Verification items for the finished model (mm, model axes). Face numbers are marked on the shaded views. A direction names the side the tool comes from. Coordinates: 2 decimals unless noted, no trailing zeros. Loops run counter-clockwise (first coordinate to the right, second up) from the corner with the lowest first, then second, coordinate; pieces in that order, holes last. Notation, with made-up numbers: (45.25, -12.5) -> (64.25, -12.5) arc R8 ccw to (64.25, -3.5) -> close; hole circle Ø9 at (29, -40). An arc over 180 degrees is marked (long way). Answer as a JSON object with one key per item and string values. Group by question number.
Q1. Cross-section at B-B on z = -4.75. Record the boundary of the cut face in (x, y) (3 decimals).
Q2. Cross-section at C-C on z = -2.75. Record the boundary of the cut face in (x, y) (3 decimals), and give its area (3 significant figures).
Q3. Scan lines: L1, parallel to X at y = 0, z = 4.05 (3 decimals); L2, parallel to X at y = 0, z = 2.5 (3 decimals); L3, parallel to X at y = 0, z = -3.95 (3 decimals). Record each from-to range of solid material in increasing order.
Q4. Set-up check for the marked faces 1, 2 and 3: record each of +Z, -Z, +X, -X, +Y, -Y from which the full face is reachable in a straight line by a thin tool's end or side.
Q5. Gauge pin test, flat ends, axial feed: pin 1 Ø4 at (y, z) = (-6, 4) entering from -X; pin 2 Ø1 at (y, z) = (-6, 1.5) entering from -X; pin 3 Ø3 at (x, y) = (8.5, 8) entering from -Z. Record the tip position at first contact, or that the pin passes through.
Q6. Release check for a two-part mould opening along Y. For the marked faces 4, 5, 6 and 7 record: released by +Y, released by -Y, zero draft, split by the parting line, or undercut.
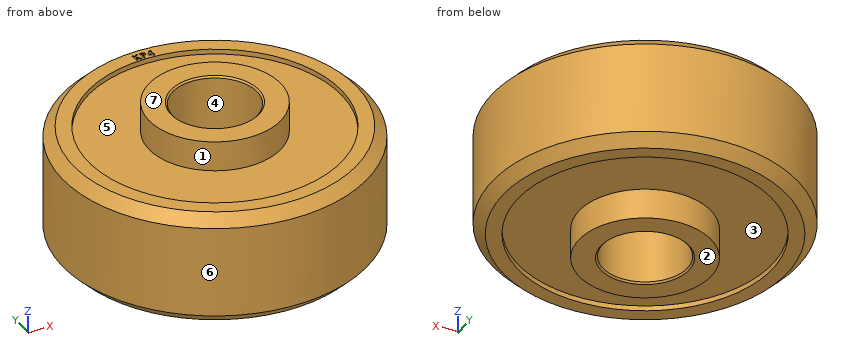
```python
from build123d import *

# Parameters (mm, degrees)
CUT_EXTRUDE1_DEPTH = 0.0635


with BuildPart() as part:
    # Sketch1 → Revolve1 (revolve)
    with BuildSketch(Plane(origin=(0, 0, 0), x_dir=(0, 0, -1), z_dir=(1, 0, 0))):
        Polygon((-6.1468, 3.302), (-6.1468, 4.953), (-3.8735, 4.953), (-3.8735, 9.525), (-4.2545, 9.525), (-4.2545, 10.63498), (-3.4417, 11.44778), (3.4417, 11.44778), (4.2545, 10.63498), (4.2545, 9.525), (3.8735, 9.525), (3.8735, 4.953), (6.1468, 4.953), (6.1468, 3.302), (6.0198, 3.175), (-6.0198, 3.175), align=None)
    revolve(axis=Axis((0, 0, 0), (0, 0, -1)))

    # Sketch2 → Cut-Extrude1 (cut)
    with BuildSketch(Plane.XY.offset(4.2545)):
        Polygon((-0.715797037, 10.256682265), (-0.59431767, 10.262024813), (-0.584777405, 10.044761191), (-0.422974521, 10.269529821), (-0.278344112, 10.275889997), (-0.486703487, 9.984593924), (-0.229243551, 9.645214917), (-0.371838703, 9.638981945), (-0.578926043, 9.910815879), (-0.566714505, 9.630459308), (-0.688193872, 9.62511676), align=None)
        with BuildLine():
            Line((-0.137056778, 10.280248194), (-0.009598846, 10.278721752))
            add(Edge.make_bspline(
                [(-0.009598846, 10.278721752), (-0.001287185, 10.278547688), (0.014749364, 10.278211849), (0.03791593, 10.277113779), (0.059251361, 10.275324059), (0.078823772, 10.273084067), (0.09658198, 10.270220031), (0.112510114, 10.266682791), (0.126614201, 10.262601864), (0.139181226, 10.258063486), (0.150404482, 10.252540227), (0.160921964, 10.246543676), (0.170857479, 10.23986336), (0.180015832, 10.232238122), (0.18873639, 10.22412794), (0.196758904, 10.215173588), (0.20416167, 10.205477286), (0.210872704, 10.195028329), (0.216953317, 10.184045094), (0.222263409, 10.172503694), (0.226470626, 10.160357095), (0.230295983, 10.147804967), (0.232853006, 10.134621192), (0.234815576, 10.120999554), (0.235807514, 10.106842586), (0.235871459, 10.09724597), (0.235903959, 10.092368587)],
                knots=[0, 0, 0, 0, 2.494e-05, 4.8119e-05, 6.9564e-05, 8.916e-05, 0.000107207, 0.000123502, 0.000138074, 0.000151235, 0.000163524, 0.000175547, 0.000187542, 0.000199383, 0.000211261, 0.000223241, 0.000235402, 0.000247822, 0.000260461, 0.000273041, 0.000285876, 0.000298999, 0.00031237, 0.000326114, 0.00034027, 0.000354901, 0.000354901, 0.000354901, 0.000354901], degree=3))
            add(Edge.make_bspline(
                [(0.235903959, 10.092368587), (0.235726012, 10.086978535), (0.235376195, 10.076382465), (0.233555914, 10.06086812), (0.230820019, 10.046045066), (0.226846103, 10.031957239), (0.221762472, 10.018597169), (0.21559979, 10.005933869), (0.208512368, 9.993900042), (0.200177911, 9.982742598), (0.191049434, 9.97230186), (0.181048202, 9.962734678), (0.170368482, 9.953924746), (0.158877942, 9.946006271), (0.146611538, 9.939059919), (0.133705365, 9.932726844), (0.119932481, 9.927410793), (0.110374057, 9.924525718), (0.105520345, 9.923060694)],
                knots=[0, 0, 0, 0, 1.6173e-05, 3.1794e-05, 4.6812e-05, 6.135e-05, 7.5642e-05, 8.9638e-05, 0.000103556, 0.000117472, 0.000131353, 0.000145118, 0.000158945, 0.000172847, 0.000186921, 0.000201201, 0.000215941, 0.000231148, 0.000231148, 0.000231148, 0.000231148], degree=3))
            add(Edge.make_bspline(
                [(0.105520345, 9.923060694), (0.102347959, 9.922302526), (0.09541168, 9.920644826), (0.084019105, 9.918830767), (0.070821383, 9.917299868), (0.055878254, 9.91624699), (0.039130219, 9.915304899), (0.020635268, 9.914885629), (0.000323735, 9.914573099), (-0.013796465, 9.914717181), (-0.021174367, 9.914792465)],
                knots=[0, 0, 0, 0, 9.782e-06, 2.1389e-05, 3.4579e-05, 4.9633e-05, 6.632e-05, 8.4899e-05, 0.000105126, 0.00012726, 0.00012726, 0.00012726, 0.00012726], degree=3))
            Line((-0.021174367, 9.914792465), (-0.024481658, 9.647283451))
            Line((-0.024481658, 9.647283451), (-0.14468899, 9.648682689))
            Line((-0.14468899, 9.648682689), (-0.137056778, 10.280248194))
        make_face()
        with BuildLine():
            Line((-0.019775128, 10.031946912), (0.01838593, 10.031438098))
            add(Edge.make_bspline(
                [(0.01838593, 10.031438098), (0.025341366, 10.031399241), (0.038074588, 10.031328107), (0.055487961, 10.032349425), (0.06951657, 10.033931542), (0.080657527, 10.0365482), (0.089494488, 10.040499929), (0.097092732, 10.045183773), (0.103672216, 10.051029279), (0.109309451, 10.057830338), (0.113976457, 10.065587683), (0.117032077, 10.074351893), (0.119207899, 10.083784291), (0.119492561, 10.090362271), (0.119639936, 10.093767826)],
                knots=[0, 0, 0, 0, 2.0862e-05, 3.8191e-05, 5.2297e-05, 6.3187e-05, 7.2357e-05, 8.1216e-05, 8.9868e-05, 9.863e-05, 0.00010764, 0.000116856, 0.000126362, 0.000136567, 0.000136567, 0.000136567, 0.000136567], degree=3))
            add(Edge.make_bspline(
                [(0.119639936, 10.093767826), (0.119562982, 10.096695704), (0.119412912, 10.102405414), (0.118359789, 10.110681571), (0.116121516, 10.118318497), (0.113057229, 10.125379216), (0.109137816, 10.131858318), (0.104301671, 10.13772663), (0.09857412, 10.142976641), (0.094159169, 10.145854249), (0.091909568, 10.14732051)],
                knots=[0, 0, 0, 0, 8.785e-06, 1.7132e-05, 2.4943e-05, 3.2576e-05, 4.0168e-05, 4.7579e-05, 5.5322e-05, 6.3367e-05, 6.3367e-05, 6.3367e-05, 6.3367e-05], degree=3))
            add(Edge.make_bspline(
                [(0.091909568, 10.14732051), (0.090027961, 10.148394937), (0.086056367, 10.150662781), (0.07913742, 10.153076263), (0.071314393, 10.15542692), (0.062261301, 10.157108271), (0.052170636, 10.158639954), (0.040923672, 10.159801584), (0.028609183, 10.160347889), (0.020039846, 10.160564391), (0.015587452, 10.16067688)],
                knots=[0, 0, 0, 0, 6.487e-06, 1.3693e-05, 2.1905e-05, 3.0986e-05, 4.1276e-05, 5.2528e-05, 6.4884e-05, 7.8245e-05, 7.8245e-05, 7.8245e-05, 7.8245e-05], degree=3))
            Line((0.015587452, 10.16067688), (-0.018248685, 10.161185694))
            Line((-0.018248685, 10.161185694), (-0.019775128, 10.031946912))
        make_face(mode=Mode.SUBTRACT)
        Polygon((0.598009372, 10.279863333), (0.718216704, 10.273375953), (0.696210494, 9.866706281), (0.752434453, 9.863653397), (0.746328683, 9.752477515), (0.690104725, 9.7555304), (0.683108531, 9.625910007), (0.565572473, 9.632270184), (0.572568667, 9.761890576), (0.296918627, 9.776773389), (0.303024397, 9.88794927), align=None)
        Polygon((0.578674437, 9.873066458), (0.590122754, 10.084733124), (0.434425638, 9.880825873), align=None, mode=Mode.SUBTRACT)
    extrude(amount=-CUT_EXTRUDE1_DEPTH, mode=Mode.SUBTRACT)


solid = part.part
```
Computed values:
{
 "1": {"outline": "circle Ø9.906 at (0, 0); hole circle Ø6.35 at (0, 0)"},
 "2": {"outline": "circle Ø22.896 at (0, 0); hole circle Ø6.35 at (0, 0)", "area": "380 mm²"},
 "3": {"L1": "x = -10.839 to -9.525, -4.953 to -3.175, 3.175 to 4.953, 9.525 to 10.839", "L2": "x = -11.448 to -3.175, 3.175 to 11.448", "L3": "x = -10.939 to -9.525, -4.953 to -3.175, 3.175 to 4.953, 9.525 to 10.939"},
 "4": {"face 1": "+Z", "face 2": "-Z, +X, -X, +Y, -Y", "face 3": "-Z"},
 "5": {"pin 1": "stops at x = -10.7", "pin 2": "stops at x = -10.04", "pin 3": "stops at z = -4.25"},
 "6": {"face 4": "undercut", "face 5": "undercut", "face 6": "split by the parting line", "face 7": "zero draft"}
}
